Geometry: final body of the model. Coordinates: model frame, mm. A direction names the side the tool comes from. Give positions to 0.01 mm unless a question says otherwise; leave off trailing zeros. Write each loop counter-clockwise with the first axis right and the second up, starting at its lowest first coordinate (ties: lowest second). Pieces come first, ordered by that corner, then holes.
Q1. Reachability of faces 4 (the flat face through (6.096, 5, 5)), 5 (the conical face through (15.24, 4.562, 2.373)) from +Z, -Z, +X, -X, +Y, -Y: full face, straight path, thin tool, end or side. Return the list, or none.
Q2. Section C-C (x = 21). Return the cut outline in (y, z), plus the area to 3 significant figures.
Q3. Mould query, pull axis Y, two halves, no side actions, for faces 1 (the cylindrical face through (11.58, -3.35, 0.74)), 2 (the cylindrical face through (19.17, -4.66, -0.61)), 3 (the flat face through (22.847, -4, -1)). Classes: +Y half, -Y half, draft (parallel to the pull), parting line (faces both ways), or undercut.
Q4. Line query: line 1 (Y direction, x = 16.75, z = 0); line 2 (Y direction, x = 20.25, z = -1.25); line 3 (Z direction, x = 22, y = -2). Output: solid intervals per line, ascending.
Q5. Pin query (flat end, axial travel): pin 1 Ø6 at (x, z) = (20, 6.5) entering from -Y; pin 2 Ø1 at (x, y) = (10, 4) entering from -Z; pin 3 Ø4 at (x, z) = (20.5, -2) entering from -Y. Return the tip coordinate at first contact, or that it passes through.
Q6. Section D-D (x = 2). Return the cut outline in (y, z).
from build123d import *
from OCP.BRepFilletAPI import BRepFilletAPI_MakeChamfer

# Parameters (mm, degrees)
SKETCH1_W          = 6.096
SKETCH1_H          = 6.858
SKETCH2_R          = 3.429
CUT_EXTRUDE1_DEPTH = 29.408287616
CHAMFER1_SIZE      = 0.254
CHAMFER1_SIZE2     = 0.181544311


with BuildPart() as part:
    # Sketch1 → Revolve1 (revolve)
    with BuildSketch(Plane.XY, mode=Mode.PRIVATE) as revolve1_sk:
        with Locations((3.048, 3.429)):
            Rectangle(SKETCH1_W, SKETCH1_H)
        Polygon((6.096, 6.858), (6.096, 0), (15.8369, 0), (15.8369, 4.699), (6.096, 11.938), align=None)
        Polygon((15.8369, 4.699), (15.8369, 0), (17.1069, 0), (18.6182, 0), (20.1295, 0), (21.3995, 0), (22.8473, 0), (22.8473, 4.699), align=None)
    revolve(revolve1_sk.sketch.rotate(Axis((6.096, 0, 0), (1, 0, 0)), 90), axis=Axis((6.096, 0, 0), (1, 0, 0)))

    # Sketch2 → Cut-Extrude1 (cut, through all)
    with BuildSketch(Plane(origin=(22.8473, 0, 0), x_dir=(0, 0, -1), z_dir=(1, 0, 0))):
        Circle(SKETCH2_R)
    extrude(amount=-CUT_EXTRUDE1_DEPTH, mode=Mode.SUBTRACT)

    # Chamfer1: one chamfer whose edges measure the first distance from different faces: ONE call of the kernel's chamfer builder (chamfer() names one face for all edges)
    chamfer1_edges_1 = [part.edges().sort_by_distance(p)[0] for p in [
        (0, 0, -6.858),
        (0, 0, 3.429),
        (22.8473, 0, 3.429),
        (22.8473, 0, -4.699),
    ]]
    chamfer1_edges_2 = [part.edges().sort_by_distance(p)[0] for p in [
        (6.096, 0, -11.938),
    ]]
    chamfer1_side_2 = [part.faces().sort_by_distance(p)[0] for p in [
        (10.96645, 0, -8.3185),
    ]]
    chamfer1 = BRepFilletAPI_MakeChamfer(part.part.solid().wrapped)
    for e in chamfer1_edges_1:
        chamfer1.Add(CHAMFER1_SIZE, e.wrapped)
    for e in chamfer1_edges_2:
        chamfer1.Add(CHAMFER1_SIZE, CHAMFER1_SIZE2, e.wrapped, chamfer1_side_2[0].wrapped)  # the first distance lies on this face
    add(Compound.cast(chamfer1.Shape()), mode=Mode.REPLACE)


solid = part.part
Computed:
1. face 4: -X
1. face 5: +X
2. outline: circle Ø9.4 at (0, 0); hole circle Ø6.86 at (0, 0)
2. area: 32.4 mm2
3. face 1: undercut
3. face 2: parting line
3. face 3: draft
4. line 1: y = -4.7 to -3.43, 3.43 to 4.7
4. line 2: y = -4.53 to -3.19, 3.19 to 4.53
4. line 3: z = -4.25 to -2.79, 2.79 to 4.25
5. pin 1: stops at y = -3.14
5. pin 2: stops at z = -8.57
5. pin 3: stops at y = -4.7
6. outline: circle Ø13.72 at (0, 0); hole circle Ø6.86 at (0, 0)
